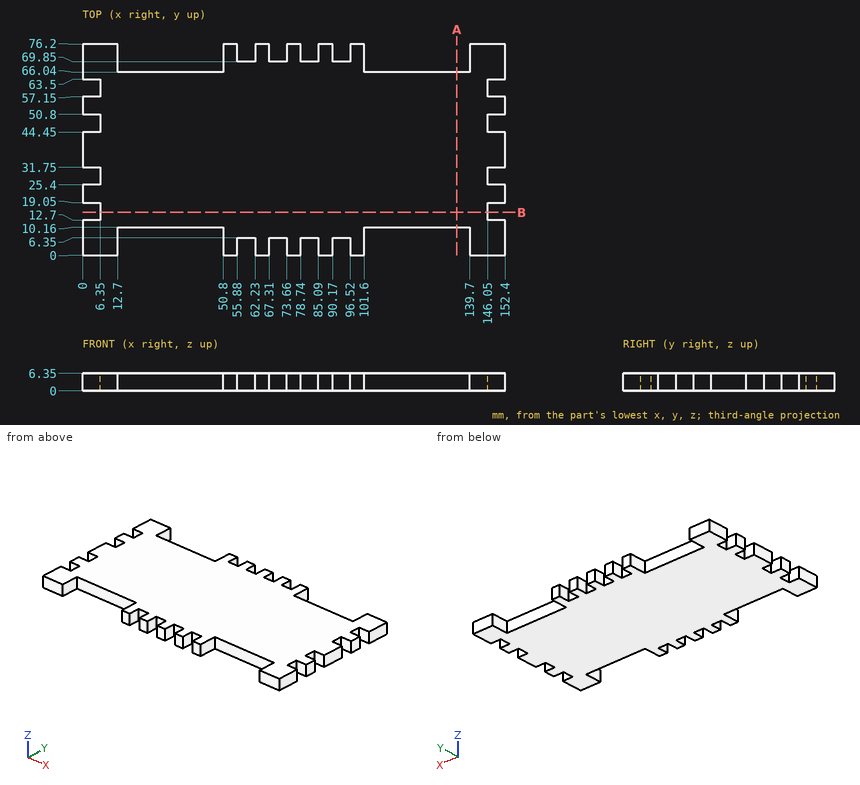
Print and shaded views of the part. All mm, measured from the part's lowest x, y and z. Round coordinates to 2 decimals unless told otherwise and drop trailing zeros. Write each loop counter-clockwise with the first axis right and the second up, starting at its lowest first coordinate (ties: lowest second). Pieces come first, ordered by that corner, then holes. Notation, with made-up numbers: (2, 3.5) - (12, 3.5) arc R18 cw to (12, 27.5) - close; hole circle Ø11 at (-24.5, 57.5). An arc over 180 degrees is marked (long way). Write each question's results on one line, items separated by ' | '. Start each with the question number.
Item 1: Saw through at A-A (x = 135). Write the cut outline in (y, z).
Item 2: Wall check: L1, parallel to X at y = 69.5, z = 0.5; L2, parallel to X at y = 57.5, z = 6; L3, parallel to Y at x = 116.5, z = 2. Give the ranges that are in metal, low to high. Write a range as [from, to].
Item 3: Saw through at B-B (y = 15.5). Write the cut outline in (x, z), and give its area (3 significant figures).
Item 4: Drop a flat-ended pin along its axis: P1, Ø3, axis at x = 134.5, z = 3, coming from the +Y side. Give the stop position or say it passes through.
Results are:
1) outline: (10.16, 0) - (66.04, 0) - (66.04, 6.35) - (10.16, 6.35) - close
2) L1: x = [0, 12.7], [50.8, 101.6], [139.7, 152.4] | L2: x = [6.35, 146.05] | L3: y = [10.16, 66.04]
3) outline: (6.35, 0) - (146.05, 0) - (146.05, 6.35) - (6.35, 6.35) - close | area: 887 mm²
4) P1: stops at y = 66.04
